Input: part model. Units: mm. Frame: model coordinates. Coordinates: 2 decimals unless noted, no trailing zeros. Loops run counter-clockwise (first coordinate to the right, second up) from the corner with the lowest first, then second, coordinate; pieces in that order, holes last. Notation, with made-up numbers: M -14,-9.75 L 23,-9.75 A3 ccw 23,-4.75 Z; hole C 1,74.25 d4. An arc over 180 degrees is marked long. Use a Markdown table: item, result. Add a question column.
1. Line query: L1, parallel to Z at x = -69, y = 0.4; L2, parallel to X at y = 0.35, z = 0; L3, parallel to Z at x = 19.5, y = 1.2. Output: solid intervals per line, ascending. Write a range as [from, to].
2. Section B-B on x = 69. Output: boundary loops of the cut face in (y, z).
3. Section C-C on x = 0. Output: boundary loops of the cut face in (y, z), then the cut area to 3 significant figures.
4. Section A-A on z = 0. Output: boundary loops of the cut face in (x, y), then the cut area to 3 significant figures.
5. Pin query (flat end, axial travel): pin 1 (1.9 mm diameter, centred on x = -32.57, z = -13.49, fed in from +Y); pin 2 (1 mm diameter, centred on y = 1, z = 53, fed in from -X); pin 3 (0.6 mm diameter, centred on x = -64, y = 1, fed in from +Z); pin 4 (5 mm diameter, centred on x = 69, z = 34, fed in from +Y). Return the tip coordinate at first contact, or that it passes through.
6. Section D-D on x = -20.5. Output: boundary loops of the cut face in (y, z).
```python
from build123d import *

# Parameters (mm, degrees)
SKETCH1_W                     = 145
SKETCH1_H                     = 132
SKETCH1_R                     = 30
BOSS_EXTRUDE1_DEPTH           = 2.032
CSK_FOR_M3_SFHCS1_AT_2_COUNT  = 2
CSK_FOR_M3_SFHCS1_AT_2_PITCH  = 26.979181982
CSK_FOR_M3_SFHCS1_AT_3_COUNT  = 2
CSK_FOR_M3_SFHCS1_AT_3_PITCH  = 49.851028074
CSK_FOR_M3_SFHCS1_AT_4_COUNT  = 2
CSK_FOR_M3_SFHCS1_AT_4_PITCH  = 65.133507042
CSK_FOR_M3_SFHCS1_AT_5_COUNT  = 2
CSK_FOR_M3_SFHCS1_AT_5_PITCH  = 70.5
CSK_FOR_M3_SFHCS1_AT_6_COUNT  = 2
CSK_FOR_M3_SFHCS1_AT_6_PITCH  = 65.133507042
CSK_FOR_M3_SFHCS1_AT_7_COUNT  = 2
CSK_FOR_M3_SFHCS1_AT_7_PITCH  = 49.851028074
CSK_FOR_M3_SFHCS1_AT_8_COUNT  = 2
CSK_FOR_M3_SFHCS1_AT_8_PITCH  = 26.979181982
CSK_FOR_M3_SFHCS2_AT_2_COUNT  = 2
CSK_FOR_M3_SFHCS2_AT_2_PITCH  = 20.506096654
CSK_FOR_M3_SFHCS2_AT_3_COUNT  = 2
CSK_FOR_M3_SFHCS2_AT_3_PITCH  = 34
CSK_FOR_M3_SFHCS2_AT_4_COUNT  = 2
CSK_FOR_M3_SFHCS2_AT_4_PITCH  = 142.126704036
CSK_FOR_M3_SFHCS2_AT_5_COUNT  = 2
CSK_FOR_M3_SFHCS2_AT_5_PITCH  = 124.348301154
CSK_FOR_M3_SFHCS2_AT_6_COUNT  = 2
CSK_FOR_M3_SFHCS2_AT_6_PITCH  = 138
CSK_FOR_M3_SFHCS2_AT_7_COUNT  = 2
CSK_FOR_M3_SFHCS2_AT_7_PITCH  = 153.844076909
CSK_FOR_M3_SFHCS2_AT_8_COUNT  = 2
CSK_FOR_M3_SFHCS2_AT_8_PITCH  = 68
CSK_FOR_M3_SFHCS2_AT_9_COUNT  = 2
CSK_FOR_M3_SFHCS2_AT_9_PITCH  = 100.713703139
CSK_FOR_M3_SFHCS2_AT_10_COUNT = 2
CSK_FOR_M3_SFHCS2_AT_10_PITCH = 115.206336631
CSK_FOR_M3_SFHCS2_AT_11_COUNT = 2
CSK_FOR_M3_SFHCS2_AT_11_PITCH = 137.58815356
CSK_FOR_M3_SFHCS2_AT_12_COUNT = 2
CSK_FOR_M3_SFHCS2_AT_12_PITCH = 155.181345528
SKETCH9_W                     = 13.5
SKETCH9_H                     = 10
CUT_EXTRUDE3_DEPTH            = 3.032
FILLET1_R                     = 1


with BuildPart() as part:
    # Sketch1 → Boss-Extrude1 (new body)
    with BuildSketch(Plane(origin=(0, 0, 0), x_dir=(1, 0, 0), z_dir=(0, 1, 0))):
        with Locations((0, 8)):
            Rectangle(SKETCH1_W, SKETCH1_H)
        Circle(SKETCH1_R, mode=Mode.SUBTRACT)
    extrude(amount=BOSS_EXTRUDE1_DEPTH)

    # Sketch2 → CSK for M3 SFHCS1 (revolve, cut)
    with BuildSketch(Plane(origin=(13.489590991, 2.032, 32.566753521), x_dir=(0, 0, 1), z_dir=(1, 0, 0))):
        Polygon((0, 0), (0, 2.032), (1.6, 2.032), (1.6, 1.4), (3, 0), align=None)
    csk_for_m3_sfhcs1 = revolve(axis=Axis((13.489590991, 8.382, 32.566753521), (0, -1, 0)), mode=Mode.SUBTRACT)

    # CSK for M3 SFHCS1 at 2: CSK for M3 SFHCS1 ×2
    with Locations(*[Vector(0.707106781, 0, -0.707106781) * (i * CSK_FOR_M3_SFHCS1_AT_2_PITCH) for i in range(1, CSK_FOR_M3_SFHCS1_AT_2_COUNT)]):
        add(csk_for_m3_sfhcs1, mode=Mode.SUBTRACT)

    # CSK for M3 SFHCS1 at 3: CSK for M3 SFHCS1 ×2
    with Locations(*[Vector(0.382683432, 0, -0.923879533) * (i * CSK_FOR_M3_SFHCS1_AT_3_PITCH) for i in range(1, CSK_FOR_M3_SFHCS1_AT_3_COUNT)]):
        add(csk_for_m3_sfhcs1, mode=Mode.SUBTRACT)

    # CSK for M3 SFHCS1 at 4: CSK for M3 SFHCS1 ×2
    with Locations(*[(0, 0, -i * CSK_FOR_M3_SFHCS1_AT_4_PITCH) for i in range(1, CSK_FOR_M3_SFHCS1_AT_4_COUNT)]):
        add(csk_for_m3_sfhcs1, mode=Mode.SUBTRACT)

    # CSK for M3 SFHCS1 at 5: CSK for M3 SFHCS1 ×2
    with Locations(*[Vector(-0.382683432, 0, -0.923879533) * (i * CSK_FOR_M3_SFHCS1_AT_5_PITCH) for i in range(1, CSK_FOR_M3_SFHCS1_AT_5_COUNT)]):
        add(csk_for_m3_sfhcs1, mode=Mode.SUBTRACT)

    # CSK for M3 SFHCS1 at 6: CSK for M3 SFHCS1 ×2
    with Locations(*[Vector(-0.707106781, 0, -0.707106781) * (i * CSK_FOR_M3_SFHCS1_AT_6_PITCH) for i in range(1, CSK_FOR_M3_SFHCS1_AT_6_COUNT)]):
        add(csk_for_m3_sfhcs1, mode=Mode.SUBTRACT)

    # CSK for M3 SFHCS1 at 7: CSK for M3 SFHCS1 ×2
    with Locations(*[Vector(-0.923879533, 0, -0.382683432) * (i * CSK_FOR_M3_SFHCS1_AT_7_PITCH) for i in range(1, CSK_FOR_M3_SFHCS1_AT_7_COUNT)]):
        add(csk_for_m3_sfhcs1, mode=Mode.SUBTRACT)

    # CSK for M3 SFHCS1 at 8: CSK for M3 SFHCS1 ×2
    with Locations(*[(-i * CSK_FOR_M3_SFHCS1_AT_8_PITCH, 0, 0) for i in range(1, CSK_FOR_M3_SFHCS1_AT_8_COUNT)]):
        add(csk_for_m3_sfhcs1, mode=Mode.SUBTRACT)

    # Sketch5 → CSK for M3 SFHCS2 (revolve, cut)
    with BuildSketch(Plane(origin=(-69, 2.032, 34), x_dir=(0, 0, 1), z_dir=(1, 0, 0))):
        Polygon((0, 0), (0, 2.032), (1.6, 2.032), (1.6, 1.4), (3, 0), align=None)
    csk_for_m3_sfhcs2 = revolve(axis=Axis((-69, 8.382, 34), (0, -1, 0)), mode=Mode.SUBTRACT)

    # CSK for M3 SFHCS2 at 2: CSK for M3 SFHCS2 ×2
    with Locations(*[Vector(0.707106781, 0, 0.707106781) * (i * CSK_FOR_M3_SFHCS2_AT_2_PITCH) for i in range(1, CSK_FOR_M3_SFHCS2_AT_2_COUNT)]):
        add(csk_for_m3_sfhcs2, mode=Mode.SUBTRACT)

    # CSK for M3 SFHCS2 at 3: CSK for M3 SFHCS2 ×2
    with Locations(*[(0, 0, -i * CSK_FOR_M3_SFHCS2_AT_3_PITCH) for i in range(1, CSK_FOR_M3_SFHCS2_AT_3_COUNT)]):
        add(csk_for_m3_sfhcs2, mode=Mode.SUBTRACT)

    # CSK for M3 SFHCS2 at 4: CSK for M3 SFHCS2 ×2
    with Locations(*[Vector(0.970964612, 0, -0.239223165) * (i * CSK_FOR_M3_SFHCS2_AT_4_PITCH) for i in range(1, CSK_FOR_M3_SFHCS2_AT_4_COUNT)]):
        add(csk_for_m3_sfhcs2, mode=Mode.SUBTRACT)

    # CSK for M3 SFHCS2 at 5: CSK for M3 SFHCS2 ×2
    with Locations(*[Vector(0.993178024, 0, 0.116607946) * (i * CSK_FOR_M3_SFHCS2_AT_5_PITCH) for i in range(1, CSK_FOR_M3_SFHCS2_AT_5_COUNT)]):
        add(csk_for_m3_sfhcs2, mode=Mode.SUBTRACT)

    # CSK for M3 SFHCS2 at 6: CSK for M3 SFHCS2 ×2
    with Locations(*[(i * CSK_FOR_M3_SFHCS2_AT_6_PITCH, 0, 0) for i in range(1, CSK_FOR_M3_SFHCS2_AT_6_COUNT)]):
        add(csk_for_m3_sfhcs2, mode=Mode.SUBTRACT)

    # CSK for M3 SFHCS2 at 7: CSK for M3 SFHCS2 ×2
    with Locations(*[Vector(0.89701211, 0, -0.442005967) * (i * CSK_FOR_M3_SFHCS2_AT_7_PITCH) for i in range(1, CSK_FOR_M3_SFHCS2_AT_7_COUNT)]):
        add(csk_for_m3_sfhcs2, mode=Mode.SUBTRACT)

    # CSK for M3 SFHCS2 at 8: CSK for M3 SFHCS2 ×2
    with Locations(*[(0, 0, -i * CSK_FOR_M3_SFHCS2_AT_8_PITCH) for i in range(1, CSK_FOR_M3_SFHCS2_AT_8_COUNT)]):
        add(csk_for_m3_sfhcs2, mode=Mode.SUBTRACT)

    # CSK for M3 SFHCS2 at 9: CSK for M3 SFHCS2 ×2
    with Locations(*[Vector(0.183689006, 0, -0.982984409) * (i * CSK_FOR_M3_SFHCS2_AT_9_PITCH) for i in range(1, CSK_FOR_M3_SFHCS2_AT_9_COUNT)]):
        add(csk_for_m3_sfhcs2, mode=Mode.SUBTRACT)

    # CSK for M3 SFHCS2 at 10: CSK for M3 SFHCS2 ×2
    with Locations(*[Vector(0.420983788, 0, -0.907068162) * (i * CSK_FOR_M3_SFHCS2_AT_10_PITCH) for i in range(1, CSK_FOR_M3_SFHCS2_AT_10_COUNT)]):
        add(csk_for_m3_sfhcs2, mode=Mode.SUBTRACT)

    # CSK for M3 SFHCS2 at 11: CSK for M3 SFHCS2 ×2
    with Locations(*[Vector(0.65049205, 0, -0.759513063) * (i * CSK_FOR_M3_SFHCS2_AT_11_PITCH) for i in range(1, CSK_FOR_M3_SFHCS2_AT_11_COUNT)]):
        add(csk_for_m3_sfhcs2, mode=Mode.SUBTRACT)

    # CSK for M3 SFHCS2 at 12: CSK for M3 SFHCS2 ×2
    with Locations(*[Vector(0.770066786, 0, -0.637963279) * (i * CSK_FOR_M3_SFHCS2_AT_12_PITCH) for i in range(1, CSK_FOR_M3_SFHCS2_AT_12_COUNT)]):
        add(csk_for_m3_sfhcs2, mode=Mode.SUBTRACT)

    # Sketch9 → Cut-Extrude3 (cut, through all)
    with BuildSketch(Plane(origin=(0, 2.032, 0), x_dir=(1, 0, 0), z_dir=(0, 1, 0))):
        with Locations((-65.75, -53)):
            Rectangle(SKETCH9_W, SKETCH9_H)
        with Locations((65.75, -53)):
            Rectangle(SKETCH9_W, SKETCH9_H)
        Polygon((-26, 74), (-59, 69.528648916), (-59, 43.5), (-72.5, 43.5), (-72.5, 74), align=None)
        Polygon((72.5, 74), (72.5, 43.5), (59, 43.5), (59, 69.528648916), (26, 74), align=None)
    extrude(amount=-CUT_EXTRUDE3_DEPTH, mode=Mode.SUBTRACT)

    # Fillet1
    fillet1_edges = [part.edges().sort_by_distance(p)[0] for p in [
        (-72.5, 1.016, 48),
        (-59, 1.016, 48),
        (-59, 1.016, 58),
        (72.5, 1.016, 48),
        (59, 1.016, 58),
        (59, 1.016, 48),
        (-59, 1.016, -69.528648916),
        (-59, 1.016, -43.5),
        (-72.5, 1.016, -43.5),
        (72.5, 1.016, -43.5),
        (59, 1.016, -43.5),
        (59, 1.016, -69.528648916),
    ]]
    fillet(fillet1_edges, radius=FILLET1_R)


solid = part.part
```
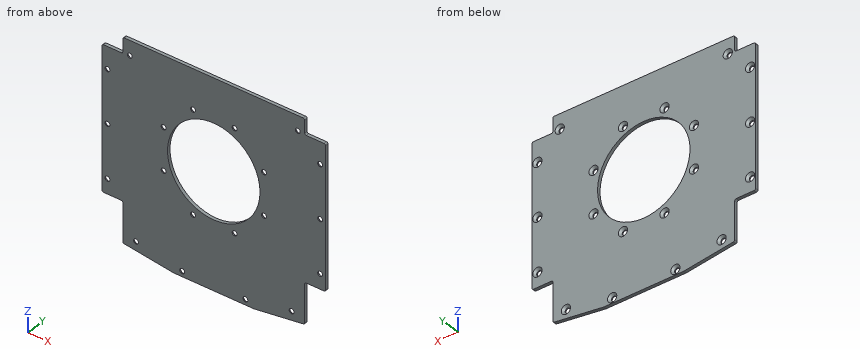
Answers below:
| question | item | result |
|---|---|---|
| 1 | L1 | z = [-43.5, -35.6], [-32.4, -1.6], [1.6, 32.4], [35.6, 48] |
| 1 | L2 | x = [-72.5, -70.6], [-67.4, -30], [30, 67.4], [70.6, 72.5] |
| 1 | L3 | z = [-74, -72.42], [-68.58, -22.8], [22.8, 58] |
| 2 | outline | M 0,-43.5 L 2.03,-43.5 L 2.03,-37 L 0.63,-35.6 L 0,-35.6 Z; M 0,-32.4 L 0.63,-32.4 L 2.03,-31 L 2.03,-3 L 0.63,-1.6 L 0,-1.6 Z; M 0,1.6 L 0.63,1.6 L 2.03,3 L 2.03,31 L 0.63,32.4 L 0,32.4 Z; M 0,35.6 L 0.63,35.6 L 2.03,37 L 2.03,48 L 0,48 Z |
| 3 | outline | M 0,-74 L 2.03,-74 L 2.03,-30 L 0,-30 Z; M 0,30 L 2.03,30 L 2.03,58 L 0,58 Z |
| 3 | area | 146 mm² |
| 4 | outline | M -72.5,0 L -70.6,0 L -70.6,0.63 L -72,2.03 L -72.5,2.03 Z; M -67.4,0 L -30,0 L -30,2.03 L -66,2.03 L -67.4,0.63 Z; M 30,0 L 67.4,0 L 67.4,0.63 L 66,2.03 L 30,2.03 Z; M 70.6,0 L 72.5,0 L 72.5,2.03 L 72,2.03 L 70.6,0.63 Z |
| 4 | area | 156 mm² |
| 5 | pin 1 | passes through |
| 5 | pin 2 | stops at x = -59 |
| 5 | pin 3 | stops at z = 48 |
| 5 | pin 4 | stops at y = 1.53 |
| 6 | outline | M 0,-74 L 2.03,-74 L 2.03,-73.5 L 0.63,-72.1 L 0,-72.1 Z; M 0,-68.9 L 0.63,-68.9 L 2.03,-67.5 L 2.03,-21.9 L 0,-21.9 Z; M 0,21.9 L 2.03,21.9 L 2.03,58 L 0,58 Z |
